```python
from build123d import *

# Parameters (mm, degrees)
F1_DEPTH = 10


with BuildPart() as f1:
    # F0 (on Front) → F1 (new body, symmetric)
    with BuildSketch(Plane.XZ):
        with BuildLine():
            Line((-35, 11.2), (-35, 15))
            ThreePointArc((-35, 15), (-53.973666, -26.278821), (-10.290488, -13.8))
            Line((-10.290488, -13.8), (0, -13.8))
            Line((0, -13.8), (0, -10))
            Line((0, -10), (-10, -10))
            Line((-10, -10), (-10, -2.5))
            ThreePointArc((-10, -2.5), (-8.94949, 0), (-10, 2.5))
            Line((-10, 2.5), (-10, 10))
            Line((-10, 10), (-13.8, 10))
            Line((-13.8, 10), (-13.8, -10))
            ThreePointArc((-13.8, -10), (-49.990664, -24.990664), (-35, 11.2))
        make_face()
        with BuildLine():
            Line((0, -10), (0, -13.8))
            Line((0, -13.8), (10.290488, -13.8))
            ThreePointArc((10.290488, -13.8), (53.973666, -26.278821), (35, 15))
            Line((35, 15), (35, 11.2))
            ThreePointArc((35, 11.2), (49.990664, -24.990664), (13.8, -10))
            Line((13.8, -10), (13.8, 10))
            Line((13.8, 10), (10, 10))
            Line((10, 10), (10, 2.5))
            ThreePointArc((10, 2.5), (8.94949, 0), (10, -2.5))
            Line((10, -2.5), (10, -10))
            Line((10, -10), (0, -10))
        make_face()
    extrude(amount=F1_DEPTH, both=True)


solid = f1.part
```
Geometry check sheet. Reference: the model listing, model coordinates, mm. A direction names the side the tool comes from. Give positions to 0.01 mm unless a question says otherwise; leave off trailing zeros. Loops run counter-clockwise (first coordinate to the right, second up) from the corner with the lowest first, then second, coordinate; pieces in that order, holes last. Notation, with made-up numbers: M 53,2 L 75,2 A12 cw 75,12 Z; hole C 21.25,55 d2. An arc over 180 degrees is marked long. Write item = value, one per line. Start each with the question number.
1. Section check A-A, the plane z = -8. Enter the section's corners in (x, y), plus the area to 3 significant figures.
2. Thickness scan on probe 1 along X at (y, z) = (-3, -5); probe 2 along X at (y, z) = (-1.5, 1); probe 3 along Z at (x, y) = (2, 6.5). Record the ranges inside material, lowest first.
3. Section check D-D, the plane z = 8.5. Enter the section's corners in (x, y).
4. Section check C-C, the plane y = 8. Enter the section's corners in (x, z).
5. Tool access check on faces 1 (the face through (-8.95, -0.14, -0.04)), 2 (the face through (-10, 0, 6)), 3 (the face through (0, 0, -13.8)). Record the directions out of +Z, -Z, +X, -X, +Y, -Y that give a thin tool (end or side, any length) a straight path to the whole face; none if there is none.
6. Section check B-B, the plane x = -49.5. Enter the section's corners in (y, z).
7. Draft check along Z on faces 4 (the face through (12, 0, 10)), 5 (the face through (-49.488, -0.14, -25.477)), 6 (the face through (-13.8, 0, 0)). Enter one of: +Z half, -Z half, draft (parallel to the pull), parting line (faces both ways), or undercut.
8. Go/stop test with flat-tipped pins: P1, Ø3, axis at y = 0.5, z = 13, coming from the -X side; P2, Ø4, axis at y = -2, z = 6.5, coming from the -X side; P3, Ø8, axis at y = 3.5, z = -5.5, coming from the -X side (3 decimals). Record where each tip stops, or that it passes through.
Values follow:
q1.outline = M -59.92,-10 L -56.11,-10 L -56.11,10 L -59.92,10 Z; M -13.8,-10 L -10,-10 L -10,10 L -13.8,10 Z; M 10,-10 L 13.8,-10 L 13.8,10 L 10,10 Z; M 56.11,-10 L 59.92,-10 L 59.92,10 L 56.11,10 Z
q1.area = 305 mm^2
q2.probe_1 = -59.49 to -55.6, -13.8 to -10, 10 to 13.8, 55.6 to 59.49
q2.probe_2 = -57.45 to -53.12, -13.8 to -9.1, 9.1 to 13.8, 53.12 to 57.45
q2.probe_3 = -13.8 to -10
q3.outline = M -51.82,-10 L -45.35,-10 L -45.35,10 L -51.82,10 Z; M -13.8,-10 L -10,-10 L -10,10 L -13.8,10 Z; M 10,-10 L 13.8,-10 L 13.8,10 L 10,10 Z; M 45.35,-10 L 51.82,-10 L 51.82,10 L 45.35,10 Z
q4.outline = M -35,11.2 L -35,15 A25 ccw long -10.29,-13.8 L 10.29,-13.8 A25 ccw long 35,15 L 35,11.2 A21.2 cw long 13.8,-10 L 13.8,10 L 10,10 L 10,2.5 A3.5 ccw 10,-2.5 L 10,-10 L -10,-10 L -10,-2.5 A3.5 ccw -10,2.5 L -10,10 L -13.8,10 L -13.8,-10 A21.2 cw long Z
q5.face_1 = +Y, -Y
q5.face_2 = +Z, +Y, -Y
q5.face_3 = -Z, +Y, -Y
q6.outline = M -10,-30.37 L 10,-30.37 L 10,-25.47 L -10,-25.47 Z; M -10,5.47 L 10,5.47 L 10,10.37 L -10,10.37 Z
q7.face_4 = +Z half
q7.face_5 = undercut
q7.face_6 = draft
q8.P1 = -47.76
q8.P2 = -55.37
q8.P3 = -59.995
